```python
from build123d import *

# Parameters (mm, degrees)
SKETCH1_W            = 66
SKETCH1_H            = 33
BOSS_EXTRUDE1_DEPTH  = 4
CUT_EXTRUDE1_DEPTH   = 5
BOSS_EXTRUDE2_DEPTH  = 20
BOSS_EXTRUDE3_DEPTH  = 1.3
BOSS_EXTRUDE4_DEPTH  = 1.3
BOSS_EXTRUDE5_DEPTH  = 1.3
BOSS_EXTRUDE6_DEPTH  = 1.3
SKETCH11_W           = 66
SKETCH11_H           = 8
CUT_EXTRUDE4_DEPTH   = 10
SKETCH13_W           = 4
SKETCH13_H           = 25
BOSS_EXTRUDE7_DEPTH  = 5
SKETCH14_W           = 4
SKETCH14_H           = 25
BOSS_EXTRUDE8_DEPTH  = 8
SKETCH16_R           = 1.75
CUT_EXTRUDE5_DEPTH   = 12
SKETCH17_R           = 1.75
CUT_EXTRUDE8_DEPTH   = 12
SKETCH18_W           = 4
SKETCH18_H           = 25
CUT_EXTRUDE9_DEPTH   = 3
SKETCH19_W           = 4
SKETCH19_H           = 25
BOSS_EXTRUDE10_DEPTH = 4
SKETCH20_W           = 4
SKETCH20_H           = 25
BOSS_EXTRUDE11_DEPTH = 20
SKETCH21_R           = 1.75
CUT_EXTRUDE10_DEPTH  = 20
SKETCH22_W           = 16
SKETCH22_H           = 25
CUT_EXTRUDE11_DEPTH  = 25


with BuildPart() as part:
    # Sketch1 → Boss-Extrude1 (new body)
    with BuildSketch(Plane.XY):
        with Locations((33, 16.5)):
            Rectangle(SKETCH1_W, SKETCH1_H)
    extrude(amount=BOSS_EXTRUDE1_DEPTH)

    # Sketch2 → Cut-Extrude1 (cut, through all)
    with BuildSketch(Plane.XY.offset(4)):
        with BuildLine():
            Line((18, 33), (48, 33))
            ThreePointArc((48, 33), (33, 18), (18, 33))
        make_face()
    extrude(amount=-CUT_EXTRUDE1_DEPTH, mode=Mode.SUBTRACT)

    # Sketch3 → Boss-Extrude2 (add)
    with BuildSketch(Plane.XY.offset(4)):
        with BuildLine():
            Line((18, 33), (15.5, 33))
            ThreePointArc((15.5, 33), (33, 15.5), (50.5, 33))
            Line((50.5, 33), (48, 33))
            ThreePointArc((48, 33), (33, 18), (18, 33))
        make_face()
    extrude(amount=BOSS_EXTRUDE2_DEPTH)

    # Sketch5 → Boss-Extrude3 (add)
    with BuildSketch(Plane.XY.offset(4.6)):
        with BuildLine():
            Line((18, 33), (21.25, 33))
            ThreePointArc((21.25, 33), (33, 21.25), (44.75, 33))
            Line((44.75, 33), (48, 33))
            ThreePointArc((48, 33), (33, 18), (18, 33))
        make_face()
    extrude(amount=BOSS_EXTRUDE3_DEPTH)

    # Sketch6 → Boss-Extrude4 (add)
    with BuildSketch(Plane.XY.offset(9.4)):
        with BuildLine():
            Line((18, 33), (21.25, 33))
            ThreePointArc((21.25, 33), (33, 21.25), (44.75, 33))
            Line((44.75, 33), (48, 33))
            ThreePointArc((48, 33), (33, 18), (18, 33))
        make_face()
    extrude(amount=BOSS_EXTRUDE4_DEPTH)

    # Sketch7 → Boss-Extrude5 (add)
    with BuildSketch(Plane.XY.offset(14.2)):
        with BuildLine():
            Line((18, 33), (21.25, 33))
            ThreePointArc((21.25, 33), (33, 21.25), (44.75, 33))
            Line((44.75, 33), (48, 33))
            ThreePointArc((48, 33), (33, 18), (18, 33))
        make_face()
    extrude(amount=BOSS_EXTRUDE5_DEPTH)

    # Sketch8 → Boss-Extrude6 (add)
    with BuildSketch(Plane.XY.offset(19)):
        with BuildLine():
            Line((18, 33), (21.25, 33))
            ThreePointArc((21.25, 33), (33, 21.25), (44.75, 33))
            Line((44.75, 33), (48, 33))
            ThreePointArc((48, 33), (33, 18), (18, 33))
        make_face()
    extrude(amount=BOSS_EXTRUDE6_DEPTH)

    # Sketch11 → Cut-Extrude4 (cut)
    with BuildSketch(Plane.XY.offset(4)):
        with Locations((33, 4)):
            Rectangle(SKETCH11_W, SKETCH11_H)
    extrude(amount=-CUT_EXTRUDE4_DEPTH, mode=Mode.SUBTRACT)

    # Sketch13 → Boss-Extrude7 (add)
    with BuildSketch(Plane.ZY):
        with Locations((2, 20.5)):
            Rectangle(SKETCH13_W, SKETCH13_H)
    extrude(amount=BOSS_EXTRUDE7_DEPTH)

    # Sketch14 → Boss-Extrude8 (add)
    with BuildSketch(Plane(origin=(66, 0, 0), x_dir=(0, 0, -1), z_dir=(1, 0, 0))):
        with Locations((-2, 20.5)):
            Rectangle(SKETCH14_W, SKETCH14_H)
    extrude(amount=BOSS_EXTRUDE8_DEPTH)

    # Sketch16 → Cut-Extrude5 (cut)
    with BuildSketch(Plane(origin=(74, 0, 0), x_dir=(0, 0, -1), z_dir=(1, 0, 0))):
        with Locations((14, 13)):
            Circle(SKETCH16_R)
    extrude(amount=-CUT_EXTRUDE5_DEPTH, mode=Mode.SUBTRACT)

    # Sketch17 → Cut-Extrude8 (cut)
    with BuildSketch(Plane.XY.offset(4)):
        with Locations((59, 13)):
            Circle(SKETCH17_R)
    extrude(amount=-CUT_EXTRUDE8_DEPTH, mode=Mode.SUBTRACT)

    # Sketch18 → Cut-Extrude9 (cut)
    with BuildSketch(Plane(origin=(74, 0, 0), x_dir=(0, 0, -1), z_dir=(1, 0, 0))):
        with Locations((-2, 20.5)):
            Rectangle(SKETCH18_W, SKETCH18_H)
    extrude(amount=-CUT_EXTRUDE9_DEPTH, mode=Mode.SUBTRACT)

    # Sketch19 → Boss-Extrude10 (add)
    with BuildSketch(Plane(origin=(71, 0, 0), x_dir=(0, 0, -1), z_dir=(1, 0, 0))):
        with Locations((-2, 20.5)):
            Rectangle(SKETCH19_W, SKETCH19_H)
    extrude(amount=BOSS_EXTRUDE10_DEPTH)

    # Sketch20 → Boss-Extrude11 (add)
    with BuildSketch(Plane(origin=(0, 0, 0), x_dir=(-1, 0, 0), z_dir=(0, 0, -1))):
        with Locations((-73, 20.5)):
            Rectangle(SKETCH20_W, SKETCH20_H)
    extrude(amount=BOSS_EXTRUDE11_DEPTH)

    # Sketch21 → Cut-Extrude10 (cut)
    with BuildSketch(Plane(origin=(75, 0, 0), x_dir=(0, 0, -1), z_dir=(1, 0, 0))):
        with Locations((12, 13)):
            Circle(SKETCH21_R)
    extrude(amount=-CUT_EXTRUDE10_DEPTH, mode=Mode.SUBTRACT)

    # Sketch22 → Cut-Extrude11 (cut, through all)
    with BuildSketch(Plane.XY.offset(4)):
        with Locations((3, 20.5)):
            Rectangle(SKETCH22_W, SKETCH22_H)
    extrude(amount=-CUT_EXTRUDE11_DEPTH, mode=Mode.SUBTRACT)


solid = part.part
```
Source: CAD feature listing. Evaluate the final solid. Frame: model axes, mm. A direction names the side the tool comes from. Give positions to 0.01 mm unless a question says otherwise; leave off trailing zeros. Order: outer loops, then holes, each group sorted by start corner. A loop starts at its lowest first (then second) coordinate and runs counter-clockwise, first axis right, second up. Notation, with made-up numbers: (32, 27) -> (77, 27) arc R5 cw to (77, 33) -> close; hole circle Ø2 at (80.25, 72.5). An arc over 180 degrees is marked (long way). Use a Markdown table: item, result.
Q1. Section D-D (x = 59). Return the cut outline in (y, z).
A:
| item | result |
|---|---|
| outline | (8, 0) -> (11.25, 0) -> (11.25, 4) -> (8, 4) -> close; (14.75, 0) -> (33, 0) -> (33, 4) -> (14.75, 4) -> close |
Q2. Section B-B (z = -12). Return the cut outline in (x, y), and give its area (3 significant figures).
A:
| item | result |
|---|---|
| outline | (71, 8) -> (75, 8) -> (75, 11.25) -> (71, 11.25) -> close; (71, 14.75) -> (75, 14.75) -> (75, 33) -> (71, 33) -> close |
| area | 86.0 mm^2 |
Q3. Pull-direction query (Z, two-part tool) for faces 1 (the face through (41, 18, 0)), 2 (the face through (73.028, 14.735, -11.772)), 3 (the face through (71, 20, -10)); classes: +Z half, -Z half, draft (parallel to the pull), parting line (faces both ways), or undercut.
A:
| item | result |
|---|---|
| face 1 | -Z half |
| face 2 | undercut |
| face 3 | draft |
Q4. Material intervals for line 1 (Z direction, x = 32, y = 20); line 2 (Y direction, x = 59, z = 1); line 3 (Z direction, x = 43.5, y = 20.25), sorted ascending. Write a range as [from, to].
A:
| item | result |
|---|---|
| line 1 | [4.6, 5.9], [9.4, 10.7], [14.2, 15.5], [19, 20.3] |
| line 2 | [8, 11.25], [14.75, 33] |
| line 3 | [0, 24] |
Q5. Section C-C (y = 13). Return the cut outline in (x, z).
A:
| item | result |
|---|---|
| outline | (11, 0) -> (57.25, 0) -> (57.25, 4) -> (11, 4) -> close; (60.75, 0) -> (71, 0) -> (71, -10.25) -> (75, -10.25) -> (75, 4) -> (60.75, 4) -> close; (71, -20) -> (75, -20) -> (75, -13.75) -> (71, -13.75) -> close |
Q6. Section A-A (z = 1.5). Return the cut outline in (x, y).
A:
| item | result |
|---|---|
| outline | (11, 8) -> (75, 8) -> (75, 33) -> (48, 33) arc R15 cw to (18, 33) -> (11, 33) -> close; hole circle Ø3.5 at (59, 13) |
Q7. Access query for faces 4 (the face through (32, 21, 9.4)), 5 (the face through (32, 21, 4.6)), 6 (the face through (32, 21, 20.3)). Directions: +Z, -Z, +X, -X, +Y, -Y. A direction counts if a zero-diameter tool reaches every point of the face in a straight line with its end or side. Return the directions, or none.
A:
| item | result |
|---|---|
| face 4 | +Y |
| face 5 | -Z, +Y |
| face 6 | +Z, +Y |
Q8. First-contact query: P1, Ø12, axis at y = 26.5, z = 17, coming from the +X side; P2, Ø12, axis at x = 36.5, y = 25, coming from the -Z side; P3, Ø6, axis at y = 17, z = 17.5, coming from the -X side; P4, Ø2, axis at y = 13, z = -12, coming from the +X side. Flat tips, straight axial feed; report the tip coordinate or a pass-through.
A:
| item | result |
|---|---|
| P1 | x = 50.49 |
| P2 | z = 4.6 |
| P3 | x = 21.28 |
| P4 | through |
